Model file for the job. Use its own axes, mm. Coordinates: 2 decimals unless noted, no trailing zeros. Order: outer loops, then holes, each group sorted by start corner. A loop starts at its lowest first (then second) coordinate and runs counter-clockwise, first axis right, second up. Notation, with made-up numbers: (50.5, 41.25) -> (96.5, 41.25) arc R15 cw to (96.5, 63.25) -> close; hole circle Ø11 at (-16.5, 41.5). An arc over 180 degrees is marked (long way). Write item = value, one per line. Start each with the question number.
Q1. Cut at C-C, the plane z = 21.5. List the corners of the cut face in (x, y).
Q2. Wall check: line 1 (X direction, y = 2.25, z = 30); line 2 (X direction, y = 2.7, z = -17); line 3 (Z direction, x = 0.5, y = 1.75). Give the ranges that are in metal, low to high. Write a range as from..to.
Q3. Cut at B-B, the plane x = -10. List the corners of the cut face in (y, z).
Q4. Cut at A-A, the plane z = -0.5. List the corners of the cut face in (x, y), plus the area to 3 significant figures.
Q5. Cut at D-D, the plane y = 2.2. Give the number of separate pieces and of enclosed holes in the cut face, plus the area to 3 significant figures.
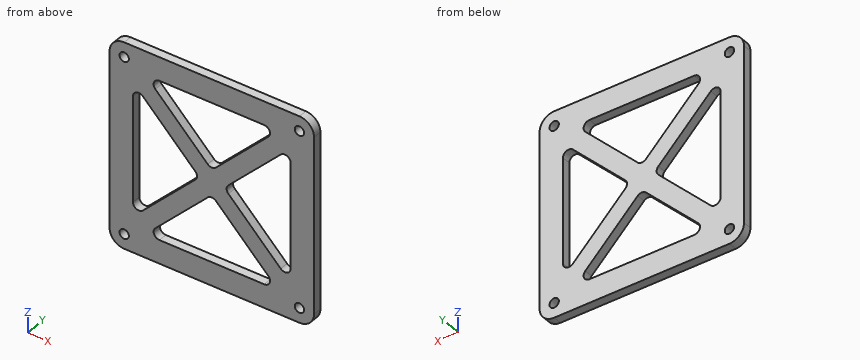
from build123d import *

# Parameters (mm, degrees)
SKETCH_1_W                       = 70
SKETCH_1_H                       = 70
SKETCH_1_R                       = 1.6
EXTRUDE_1_DEPTH                  = 3
FILLET_1_R                       = 5
CUT_EXTRUDE_2_DEPTH              = 50.588305073
FILLET_2_R                       = 2
PATTERN_CIRCULAR_1_COUNT         = 4
FILLET_2_OF_PATTERN_CIRCULAR_1_R = 2


with BuildPart() as part:
    # 草图1 → 凸台-拉伸1 (new body)
    with BuildSketch(Plane(origin=(0, 0, 0), x_dir=(1, 0, 0), z_dir=(0, 1, 0))):
        Rectangle(SKETCH_1_W, SKETCH_1_H)
        with Locations(Location((-30, 30, 0), (0, 0, 270))):
            Circle(SKETCH_1_R, mode=Mode.SUBTRACT)
        with Locations(Location((30, 30, 0), (0, 0, 270))):
            Circle(SKETCH_1_R, mode=Mode.SUBTRACT)
        with Locations(Location((30, -30, 0), (0, 0, 270))):
            Circle(SKETCH_1_R, mode=Mode.SUBTRACT)
        with Locations(Location((-30, -30, 0), (0, 0, 270))):
            Circle(SKETCH_1_R, mode=Mode.SUBTRACT)
    extrude(amount=EXTRUDE_1_DEPTH)

    # 圆角1
    fillet_1_edges = [part.edges().sort_by_distance(p)[0] for p in [
        (-35, 1.5, -35),
        (35, 1.5, -35),
        (35, 1.5, 35),
        (-35, 1.5, 35),
    ]]
    fillet(fillet_1_edges, radius=FILLET_1_R)

    # 草图2 → 切除-拉伸2 (cut, through all)
    with BuildSketch(Plane(origin=(0, 3, 0), x_dir=(1, 0, 0), z_dir=(0, 1, 0))):
        Polygon((-22.757359313, 27), (0, 4.242640687), (22.757359313, 27), align=None)
    cut_extrude_2 = extrude(amount=-CUT_EXTRUDE_2_DEPTH, mode=Mode.SUBTRACT)

    # 圆角2
    fillet_2_edges = [part.edges().sort_by_distance(p)[0] for p in [
        (22.757359313, 1.5, -27),
        (0, 1.5, -4.242640687),
        (-22.757359313, 1.5, -27),
    ]]
    fillet(fillet_2_edges, radius=FILLET_2_R)

    # 阵列(圆周)1: 切除-拉伸2 ×4 about axis
    pattern_circular_1_axis = Axis((0, 0, 0), (0, 1, 0))
    for i in range(1, PATTERN_CIRCULAR_1_COUNT):
        add(cut_extrude_2.rotate(pattern_circular_1_axis, i * 360 / PATTERN_CIRCULAR_1_COUNT), mode=Mode.SUBTRACT)

    # 圆角2 of 阵列(圆周)1
    fillet_2_of_pattern_circular_1_edges = [part.edges().sort_by_distance(p)[0] for p in [
        (-27, 1.5, -22.757359313),
        (-4.242640687, 1.5, 0),
        (-27, 1.5, 22.757359313),
        (-22.757359313, 1.5, 27),
        (0, 1.5, 4.242640687),
        (22.757359313, 1.5, 27),
        (27, 1.5, 22.757359313),
        (4.242640687, 1.5, 0),
        (27, 1.5, -22.757359313),
    ]]
    fillet(fillet_2_of_pattern_circular_1_edges, radius=FILLET_2_OF_PATTERN_CIRCULAR_1_R)


solid = part.part
Here are the results:
q1.outline = (-35, 0) -> (-17.26, 0) -> (-17.26, 3) -> (-35, 3) -> close; (17.26, 0) -> (35, 0) -> (35, 3) -> (17.26, 3) -> close
q2.line_1 = -35..-31.6, -28.4..28.4, 31.6..35
q2.line_2 = -35..-27, -21.24..-12.76, 12.76..21.24, 27..35
q2.line_3 = -35..-27, -5.13..5.13, 27..35
q3.outline = (0, -35) -> (3, -35) -> (3, -27) -> (0, -27) -> close; (0, -14.24) -> (3, -14.24) -> (3, -5.76) -> (0, -5.76) -> close; (0, 5.76) -> (3, 5.76) -> (3, 14.24) -> (0, 14.24) -> close; (0, 27) -> (3, 27) -> (3, 35) -> (0, 35) -> close
q4.outline = (-35, 0) -> (-27, 0) -> (-27, 3) -> (-35, 3) -> close; (-5.13, 0) -> (5.13, 0) -> (5.13, 3) -> (-5.13, 3) -> close; (27, 0) -> (35, 0) -> (35, 3) -> (27, 3) -> close
q4.area = 78.8 mm²
q5.separate_pieces = 1
q5.enclosed_holes = 8
q5.area = 2,820 mm²
